Could you check a few things on this model? Use its own coordinates, in mm. A direction names the side the tool comes from. Give positions to 0.01 mm unless a question says otherwise; leave off trailing zeros. Loops run counter-clockwise (first coordinate to the right, second up) from the corner with the lowest first, then second, coordinate; pieces in that order, holes last. Notation, with made-up numbers: M 75,-34.75 L 119,-34.75 A18 ccw 119,-6.75 Z; hole C -32,49 d7. An arc over 180 degrees is marked long. Use CSV: the item, a comma, the result in double quotes.
```python
from build123d import *

# Parameters (mm, degrees)
SKETCH1_R           = 9.75
BOSS_EXTRUDE1_DEPTH = 10
SKETCH5_W           = 1
SKETCH5_H           = 1


with BuildPart() as part:
    # Sketch1 → Boss-Extrude1 (new body)
    with BuildSketch(Plane(origin=(0, 0, 0), x_dir=(1, 0, 0), z_dir=(0, 1, 0))):
        with Locations(Location((0, 0, 0), (0, 0, 270))):
            Circle(SKETCH1_R)
    extrude(amount=BOSS_EXTRUDE1_DEPTH)

    # Sketch2 → Revolve1 (revolve)
    with BuildSketch(Plane.XY, mode=Mode.PRIVATE) as revolve1_sk:
        Polygon((0, 10), (0, 19.300191168), (9.75, 10), align=None)
    revolve(revolve1_sk.sketch.rotate(Axis((0, 0, 0), (0, 1, 0)), 90), axis=Axis((0, 0, 0), (0, 1, 0)))

    # Sketch3 → Cut-Revolve1 (revolve, cut)
    with BuildSketch(Plane.XY, mode=Mode.PRIVATE) as cut_revolve1_sk:
        Polygon((0, 19.300191168), (0, 19.050191168), (0.262091387, 19.050191168), align=None)
    revolve(cut_revolve1_sk.sketch.rotate(Axis((0, 19.050191168, 0), (0, 1, 0)), 90), axis=Axis((0, 19.050191168, 0), (0, 1, 0)), mode=Mode.SUBTRACT)

    # Sketch4 → Revolve2 (revolve)
    with BuildSketch(Plane.XY, mode=Mode.PRIVATE) as revolve2_sk:
        with BuildLine():
            Line((0, 19.050191168), (0, 19.300191168))
            add(Edge.make_bspline(
                [(0, 19.300191168), (0.070360222, 19.286498468), (0.134000153, 19.189472435), (0.262091387, 19.050191168)],
                knots=[0.5, 0.5, 0.5, 0.5, 1, 1, 1, 1], degree=3))
            Line((0.262091387, 19.050191168), (0, 19.050191168))
        make_face()
    revolve(revolve2_sk.sketch.rotate(Axis((0, 19.050191168, 0), (0, -1, 0)), 270), axis=Axis((0, 19.050191168, 0), (0, -1, 0)))

    # Sketch5 → Cut-Revolve2 (revolve, cut)
    with BuildSketch(Plane.XY, mode=Mode.PRIVATE) as cut_revolve2_sk:
        with Locations((-9.25, 5)):
            Rectangle(SKETCH5_W, SKETCH5_H)
    revolve(cut_revolve2_sk.sketch.rotate(Axis((0, 0, 0), (0, 1, 0)), 270), axis=Axis((0, 0, 0), (0, 1, 0)), mode=Mode.SUBTRACT)


solid = part.part
```
1. I'm going to push flat-ended pins straight in: pin 1 Ø1 at (y, z) = (8, 1.5) entering from -X; pin 2 Ø3 at (y, z) = (12.5, 3) entering from -X; pin 3 Ø5 at (y, z) = (3.5, -7.5) entering from +X. Where does each tip first touch, or does it pass through?
Outcome:
pin 1,"x = -9.7"
pin 2,"x = -8.24"
pin 3,"x = 8.37"
2. I want a section at A-A, the plane y = 10.75. List the corners of the cut face in (x, z) for me.
Outcome:
outline,"C 0,0 d17.93"
3. Which directions (+Z, -Z, +X, -X, +Y, -Y) give clear straight access to the entire face, cutting with the end or side of a thin tool? Please do faces 5 (the face through (9.667, 7.719, -1.269)), 6 (the face through (-4, 4.5, 8)).
Outcome:
face 5,"+Y, -Y"
face 6,"none"
4. I want a section at B-B, the plane y = 13.5. List the corners of the cut face in (x, z) for me, then the cut area to 3 significant figures.
Outcome:
outline,"C 0,0 d12.16"
area,"116 mm2"
5. If we mould it in two halves opening along Y, with no side actions, what happens to faces 1 (the face through (-4, 5.5, 8)), 2 (the face through (9.667, 2.218, -1.269)), 3 (the face through (0, 0, 0)), 4 (the face through (1.864, 17.478, 0.414))? For each: +Y half, -Y half, draft (parallel to the pull), parting line (faces both ways), or undercut.
Outcome:
face 1,"undercut"
face 2,"draft"
face 3,"-Y half"
face 4,"+Y half"
6. Please list where these lines run through material, in increasing order: line 1 (X direction, y = 8.25, z = 0.25); line 2 (Y direction, x = -7.75, z = -4.25); line 3 (Z direction, x = 1.5, y = 2).
Outcome:
line 1,"-9.75 to 9.75"
line 2,"0 to 4.5, 5.5 to 10.87"
line 3,"-9.63 to 9.63"
